Read the model definition and answer for the solid it produces. Units are mm, in the model's axes. A direction names the side the tool comes from. Coordinates: 2 decimals unless noted, no trailing zeros. Loops run counter-clockwise (first coordinate to the right, second up) from the corner with the lowest first, then second, coordinate; pieces in that order, holes last. Notation, with made-up numbers: (61, 53.5) - (98, 53.5) arc R19 cw to (98, 73.5) - close; hole circle Ø6 at (45, -13.75). An arc over 180 degrees is marked (long way). Use CSV: the item, a comma, the result in double quotes.
Autodesk Inventor part; units mm, degrees
ref_plane "YZ Plane" through (0, 0, 0) normal (1, 0, 0) x (0, 1, 0)
ref_plane "XZ Plane" through (0, 0, 0) normal (0, 1, 0) x (-1, 0, 0)
ref_plane "XY Plane" through (0, 0, 0) normal (0, 0, 1) x (1, 0, 0)
sketch "Sketch1" plane through (0, 0, 0) normal (0, 0, 1) x (1, 0, 0)
  circle A0 centre (5.881, 13.6671) radius 3.1287
  circle A1 centre (20.5836, 13.6671) radius 3.1287
  line L0 (0, -0.9379) -> (26.4647, -0.9379)
  line L1 (26.4647, 28.2721) -> (26.4647, -0.9379)
  line L2 (0, 28.2721) -> (26.4647, 28.2721)
  line L3 (0, -0.9379) -> (0, 28.2721)
  point P0 (0, 0)
  dimension "d4" = 14.7026
  dimension "d5" = 29.21
  dimension "d21" = 14.605
extrude "Plate1" add sketch "Sketch1" along normal blind 3.175 contours A0 | A1 | L3 L2 L1 L0
sketch "Sketch2" plane through (0, 29.5421, 4.445) normal (0, 1, 0) x (-1, 0, 0)
  line L0 (-26.4647, 0) -> (0, 0)
  line L1 (0, 0) -> (0, 20.955)
  line L2 (0, 20.955) -> (-26.4647, 20.955)
  line L3 (-26.4647, 20.955) -> (-26.4647, 0)
edge flange "Flange1" height 25.4 angle 90 thickness 3.175 bend radius 1.27 thickness toward (0, 1, 0) relief straight relief width 3.175 relief depth 1.5875 corner gap 3.175 corner form 0 edges at (13.2323, 28.2721, 3.175) (13.2323, -0.9379, 3.175) wall of the first edge with corners at (26.4647, 29.5421, 4.445) (0, 29.5421, 4.445) (0, 29.5421, 25.4) (26.4647, 29.5421, 25.4)
bend "Bend1"
corner "Corner1"
sketch "Sketch3" plane through (0, 32.7171, 25.4) normal (0, 1, 0) x (1, 0, 0)
  line L0 (26.4647, 0) -> (0, 0)
  line L1 (26.4647, 20.955) -> (26.4647, 0)
  line L2 (13.2323, 0) -> (13.2323, 6.35)
  circle A0 centre (13.2323, 6.35) radius 2.3813
  point P0 (0, 25.4)
  dimension "d17" = 6.35
  dimension "d18" = 4.7625
extrude "Extrusion1" cut sketch "Sketch3" against normal blind 76174.6
sketch "Sketch5" plane through (0, 0, 3.175) normal (0, 0, 1) x (1, 0, 0)
  circle A0 centre (20.1147, 14.1734) radius 3.3782
  circle A1 centre (4.2397, 14.1734) radius 3.3782
  point P0 (0, 0)
extrude "Cut1" cut sketch "Sketch5" against normal blind 3.175
equation "\"d22\" = Thickness"
equation "\"d7\" = BendReliefWidth"
equation "\"d8\" = BendReliefDepth"
equation "\"d9\" = MinimumRemnant"
equation "\"d10\" = BendRadius"
equation "\"d14\" = CornerReliefSize"
equation "\"d15\" = GapSize"
equation "\"d16\" = JacobiRadiusSize"
equation "\"BendRadius\" = Thickness"
equation "\"BendReliefWidth\" = Thickness"
equation "\"BendReliefDepth\" = 0.5 * Thickness"
equation "\"CornerReliefSize\" = 4 * Thickness"
equation "\"MinimumRemnant\" = 2 * Thickness"
equation "\"TransitionRadius\" = BendRadius"
equation "\"JacobiRadiusSize\" = Thickness"
equation "\"GapSize\" = Thickness"
equation "\"d6\" = BendRadius"
properties part number "pulley mount. actual ipt" material "Aluminum 6061"
Q1. Find the intervals of material crossed by probe 1 along Y at (x, z) = (1.5, 6.75); probe 2 along Z at (x, y) = (9.25, 21.5) (3 decimals); probe 3 along X at (y, z) = (31.35, 19.05), in increasing order. Write a range as [from, to].
Reported:
probe 1,"y = [-5.38, -2.21], [29.54, 32.72]"
probe 2,"z = [0, 3.175]"
probe 3,"x = [0, 10.85], [15.61, 26.46]"
Q2. Given P1, Ø4, axis at x = 20, y = 8.5, coming from the +Z side (3 decimals), flat-ended and moving along its own axis, determine where the tip first touches the part or whether it passes through.
Reported:
P1,"stops at z = 3.175"
Q3. The part is cut by section C-C on z = 19.05. Determine the outline of the cut face in (x, y).
Reported:
outline,"(0, -5.38) - (10.85, -5.38) - (10.85, -2.21) - (0, -2.21) - close; (0, 29.54) - (10.85, 29.54) - (10.85, 32.72) - (0, 32.72) - close; (15.61, -5.38) - (26.46, -5.38) - (26.46, -2.21) - (15.61, -2.21) - close; (15.61, 29.54) - (26.46, 29.54) - (26.46, 32.72) - (15.61, 32.72) - close"
Q4. A tool of negligible diameter and unlimited length cuts with its end or side. For faces 5 (the face through (13, 14, 0)), 6 (the face through (13.047, 29.18, 3.557)), from which of +Z, -Z, +X, -X, +Y, -Y can it reach the whole face along a straight path? Write none if from no direction.
Reported:
face 5,"-Z, +X, -X, +Y, -Y"
face 6,"+Z, +X, -X"
Q5. The part is cut by section B-B on x = 5.75. Determine the outline of the cut face in (y, z) (3 decimals).
Reported:
outline,"(-5.383, 4.445) arc R4.445 ccw to (-0.938, 0) - (11.152, 0) - (11.152, 3.175) - (-0.938, 3.175) arc R1.27 cw to (-2.208, 4.445) - (-2.208, 25.4) - (-5.383, 25.4) - close; (17.195, 0) - (28.272, 0) arc R4.445 ccw to (32.717, 4.445) - (32.717, 25.4) - (29.542, 25.4) - (29.542, 4.445) arc R1.27 cw to (28.272, 3.175) - (17.195, 3.175) - close"
Q6. The part is cut by section D-D on x = 14. Determine the outline of the cut face in (y, z) (3 decimals), and give its area (3 significant figures).
Reported:
outline,"(-5.383, 4.445) arc R4.445 ccw to (-0.938, 0) - (28.272, 0) arc R4.445 ccw to (32.717, 4.445) - (32.717, 16.796) - (29.542, 16.796) - (29.542, 4.445) arc R1.27 cw to (28.272, 3.175) - (-0.938, 3.175) arc R1.27 cw to (-2.208, 4.445) - (-2.208, 16.796) - (-5.383, 16.796) - close; (-5.383, 21.304) - (-2.208, 21.304) - (-2.208, 25.4) - (-5.383, 25.4) - close; (29.542, 21.304) - (32.717, 21.304) - (32.717, 25.4) - (29.542, 25.4) - close"
area,"226 mm²"
Q7. The part is cut by section A-A on z = 5.25. Determine the outline of the cut face in (x, y).
Reported:
outline,"(0, -5.38) - (26.46, -5.38) - (26.46, -2.21) - (0, -2.21) - close; (0, 29.54) - (26.46, 29.54) - (26.46, 32.72) - (0, 32.72) - close"
Q8. For a pull along Y with two mould halves and no side action, classify faces 1 (the face through (13, -5.383, 15)), 2 (the face through (13.42, -1.85, 3.56)), 3 (the face through (13, -4, 25.4)), 4 (the face through (13.047, 31.45, 1.337)) as +Y half, -Y half, draft (parallel to the pull), parting line (faces both ways), or undercut.
Reported:
face 1,"-Y half"
face 2,"undercut"
face 3,"draft"
face 4,"+Y half"
